Autodesk Inventor part; units mm, degrees
ref_plane "YZ Plane" through (0, 0, 0) normal (1, 0, 0) x (0, 1, 0)
ref_plane "XZ Plane" through (0, 0, 0) normal (0, 1, 0) x (-1, 0, 0)
ref_plane "XY Plane" through (0, 0, 0) normal (0, 0, 1) x (1, 0, 0)
sketch "Sketch1" plane through (0, 0, 0) normal (0, 0, 1) x (1, 0, 0)
  arc A0 (1.9783, 3.4766) -> (3.9987, 0.1008) centre (0, 0) ccw
  arc A1 (87.0013, 0.1008) -> (89.0217, 3.4766) centre (91, 0) ccw
  line L0 (0, 0) -> (109, 0) construction
  line L1 (8, -1.8544) -> (8, -3.8544)
  line L2 (83, -1.8544) -> (83, -3.8544)
  line L3 (45.5, 0) -> (45.5, -69) construction
  line L4 (12.5, -5.7261) -> (12.5, -7.7261)
  line L5 (78.5, -5.7261) -> (78.5, -7.7261)
  line L6 (18, -9.6033) -> (18, -11.6033)
  line L7 (73, -9.6033) -> (73, -11.6033)
  line L8 (23.5, -13.0781) -> (23.5, -15.0781)
  line L9 (67.5, -13.0781) -> (67.5, -15.0781)
  line L10 (28.5, -16.0985) -> (28.5, -18.0985)
  line L11 (62.5, -16.0985) -> (62.5, -18.0985)
  line L12 (32.5, -18.7085) -> (32.5, -20.7085)
  line L13 (58.5, -18.7085) -> (58.5, -20.7085)
  circle A2 centre (91, 0) radius 2
  circle A3 centre (0, 0) radius 2
  line L14 (38, -6.0391) -> (53, -6.0391)
  line L15 (53, -6.0391) -> (53, -24.0391)
  line L16 (53, -24.0391) -> (38, -24.0391)
  line L17 (38, -24.0391) -> (38, -6.0391)
  arc A4 (3.9987, 0.1008) -> (38, -9.726) centre (45.5, 79.9609) ccw
  arc A5 (53, -9.726) -> (87.0013, 0.1008) centre (45.5, 79.9609) ccw
  line L18 (0, -8.0391) -> (38, -8.0391) construction
  line L19 (53, -8.0391) -> (95.0831, -8.0391) construction
  arc A6 (1.9783, 3.4766) -> (38, -7.7189) centre (45.5, 79.9609) ccw
  arc A7 (53, -7.7189) -> (89.0217, 3.4766) centre (45.5, 79.9609) ccw
  arc A8 (8, -3.8544) -> (38, -11.5542) centre (45.5, 79.9609) ccw
  arc A9 (53, -11.5542) -> (83, -3.8544) centre (45.5, 79.9609) ccw
  arc A10 (12.5, -7.7261) -> (38, -13.4294) centre (45.5, 79.9609) ccw
  arc A11 (53, -13.4294) -> (78.5, -7.7261) centre (45.5, 79.9609) ccw
  arc A12 (18, -11.6033) -> (38, -15.3492) centre (45.5, 79.9609) ccw
  arc A13 (53, -15.3492) -> (73, -11.6033) centre (45.5, 79.9609) ccw
  arc A14 (23.5, -15.0781) -> (38, -17.3025) centre (45.5, 79.9609) ccw
  arc A15 (53, -17.3025) -> (67.5, -15.0781) centre (45.5, 79.9609) ccw
  arc A16 (28.5, -18.0985) -> (38, -19.2782) centre (45.5, 79.9609) ccw
  arc A17 (53, -19.2782) -> (62.5, -18.0985) centre (45.5, 79.9609) ccw
  arc A18 (32.5, -20.7085) -> (38, -21.267) centre (45.5, 79.9609) ccw
  arc A19 (53, -21.267) -> (58.5, -20.7085) centre (45.5, 79.9609) ccw
  dimension "d53" = 15
  dimension "d1" = 8
  dimension "d2" = 91
  dimension "d10" = 2
  dimension "d11" = 2
  dimension "d13" = 45.5
  dimension "d16" = 2
  dimension "d17" = 2
  dimension "d19" = 33
  dimension "d20" = 37.5
  dimension "d21" = 2
  dimension "d22" = 2
  dimension "d23" = 27.5
  dimension "d24" = 27.5
  dimension "d25" = 2
  dimension "d26" = 2
  dimension "d27" = 22
  dimension "d29" = 2
  dimension "d30" = 2
  dimension "d32" = 17
  dimension "d33" = 2
  dimension "d34" = 2
  dimension "d35" = 13
  dimension "d37" = 4
  dimension "d38" = 4
  dimension "d52" = 18
  dimension "d54" = 7.5
extrude "Extrusion5" add sketch "Sketch1" along normal mid plane 14 contours L17 L14 L15 L16
extrude "Extrusion6" add sketch "Sketch1" along normal mid plane 9 contours A6 L17 A4 A0 | A4 L17 A8 L1 | L17 A10 L4 A8 | L17 A12 L6 A10 | A7 A1 A5 L15 | L17 A14 L8 A12 | A5 L2 A9 L15 | L17 A16 L10 A14 | A9 L5 A11 L15 | L17 A18 L12 A16 | A11 L7 A13 L15 | A13 L9 A15 L15 | A15 L11 A17 L15 | A17 L13 A19 L15
sketch "Sketch2" plane through (38, -24.0391, 7) normal (0, -1, 0) x (1, 0, 0)
  circle A0 centre (7.5, -7) radius 4
  line L0 (15, -14) -> (0, -14)
  line L1 (0, -14) -> (0, 0)
  point P0 (-38, -7)
  dimension "d59" = 8
  dimension "d60" = 7
  dimension "d61" = 7.5
hole "Hole1" at (45.5, -24.0391, 0) direction (0, 1, 0) diameter 8 depth 11.72
equation "\"d19\" = d18"
equation "\"d32\" = d31"
properties part number "HUDSON-1-09-LEAF SPRING PACK"
CAD build for the part. Positions are in the model's coordinates, mm. A direction names the side the tool comes from. Round coordinates to 2 decimals unless told otherwise and drop trailing zeros. Write each loop counter-clockwise with the first axis right and the second up, starting at its lowest first coordinate (ties: lowest second). Pieces come first, ordered by that corner, then holes. Notation, with made-up numbers: M -26,33 L 25,33 A31 cw 25,62 Z; hole C 27.25,-37.75 d11. An arc over 180 degrees is marked long. One line per question, with ' | ' between items.
1. Pin check, flat tips, straight feed: pin 1 Ø1 at (x, z) = (31.5, -1.5) entering from +Y; pin 2 Ø0.6 at (y, z) = (-11, -1) entering from +X; pin 3 Ø7 at (x, z) = (45.5, 0) entering from -Y; pin 4 Ø3 at (x, y) = (0, 0) entering from -Z. Stop position of each tip, or through.
Working result:
pin 1: y = -6.84 | pin 2: x = 73 | pin 3: y = -12.32 | pin 4: through
2. Cut at D-D on z = 0. Count the separate pieces of the cut face and the enclosed holes in it, and give its area (3 significant figures).
Working result:
separate pieces: 1 | enclosed holes: 2 | area: 803 mm2
3. Probe L1, parallel to X at y = -16.75, z = 0; L2, parallel to Y at x = 0, z = -0.75; L3, parallel to Z at x = 45.5, y = -20.5. List the from-to ranges inside material, lowest first. Write a range as from..to.
Working result:
L1: 28.5..41.5, 49.5..62.5 | L2: -4..-2, 2..4 | L3: -7..-4, 4..7
4. Which spindle directions (+Z, -Z, +X, -X, +Y, -Y) get a long thin tool onto all of the face, cutting with end or side? Do faces 1 (the cylindrical face through (19.636, -4.153, -0.063)), 2 (the flat face through (69, -9, -4.5)), 3 (the flat face through (62.5, -17, 0)), 4 (the flat face through (32.5, -20, 0)). Say none if no direction does.
Working result:
face 1: +Z, -Z, +Y | face 2: -Z, +X, +Y, -Y | face 3: +Z, -Z, +X, -Y | face 4: +Z, -Z, -X, -Y
5. Cut at B-B on x = 45.5. Write the cut outline in (y, z), and give its area (3 significant figures).
Working result:
outline: M -24.04,-7 L -6.04,-7 L -6.04,7 L -24.04,7 L -24.04,4 L -12.32,4 L -12.32,-4 L -24.04,-4 Z | area: 158 mm2
6. Cut at A-A on x = 91. Write the cut outline in (y, z).
Working result:
outline: M -4,-4.5 L -2,-4.5 L -2,4.5 L -4,4.5 Z; M 2,-4.5 L 4,-4.5 L 4,4.5 L 2,4.5 Z
